Geometry check sheet. Reference: drawing and pictorial views, mm from the part's lowest x, y, z. A direction names the side the tool comes from. Give positions to 0.01 mm unless a question says otherwise; leave off trailing zeros. Write each loop counter-clockwise with the first axis right and the second up, starting at its lowest first coordinate (ties: lowest second). Pieces come first, ordered by that corner, then holes. Notation, with made-up numbers: (11.5, -18) -> (32.5, -18) arc R15 ccw to (32.5, -9) -> close; hole circle Ø1 at (19, 79). An arc over 180 degrees is marked (long way). Use a Markdown table: item, result. Add a question column.
1. Set-up check for the marked faces 4, 5 and 6: record each of +Z, -Z, +X, -X, +Y, -Y from which the full face is reachable in a straight line by a thin tool's end or side.
2. Cross-section at D-D (y = 5.5). Count the separate pieces of the cut face and the enclosed holes in it, then the cut area to 3 significant figures.
3. Release check for a two-part mould opening along X. For the marked faces 1, 2 and 3 record: released by +X, released by -X, zero draft, split by the parting line, or undercut.
4. Cross-section at C-C (x = 11). Enter the section's corners in (y, z), then the cut area to 3 significant figures.
5. Scan lines: probe 1 along X at (y, z) = (2, 1.5); probe 2 along Z at (x, y) = (44, 14.25); probe 3 along Y at (x, z) = (8, 13). Record each from-to range of solid material in increasing order. Write a range as [from, to].
6. Cross-section at A-A (z = 11). Enter the section's corners in (x, y).
7. Cross-section at B-B (y = 12.25). Enter the section's corners in (x, z).
8. Gauge pin test, flat ends, axial feed: P1, Ø7, axis at x = 23.38, z = 10.99, coming from the +Y side; P2, Ø2.5, axis at y = 15.5, z = 11.5, coming from the -X side; P3, Ø1.5, axis at x = 13, y = 17, coming from the +Z side. Record the tip position at first contact, or that the pin passes through.
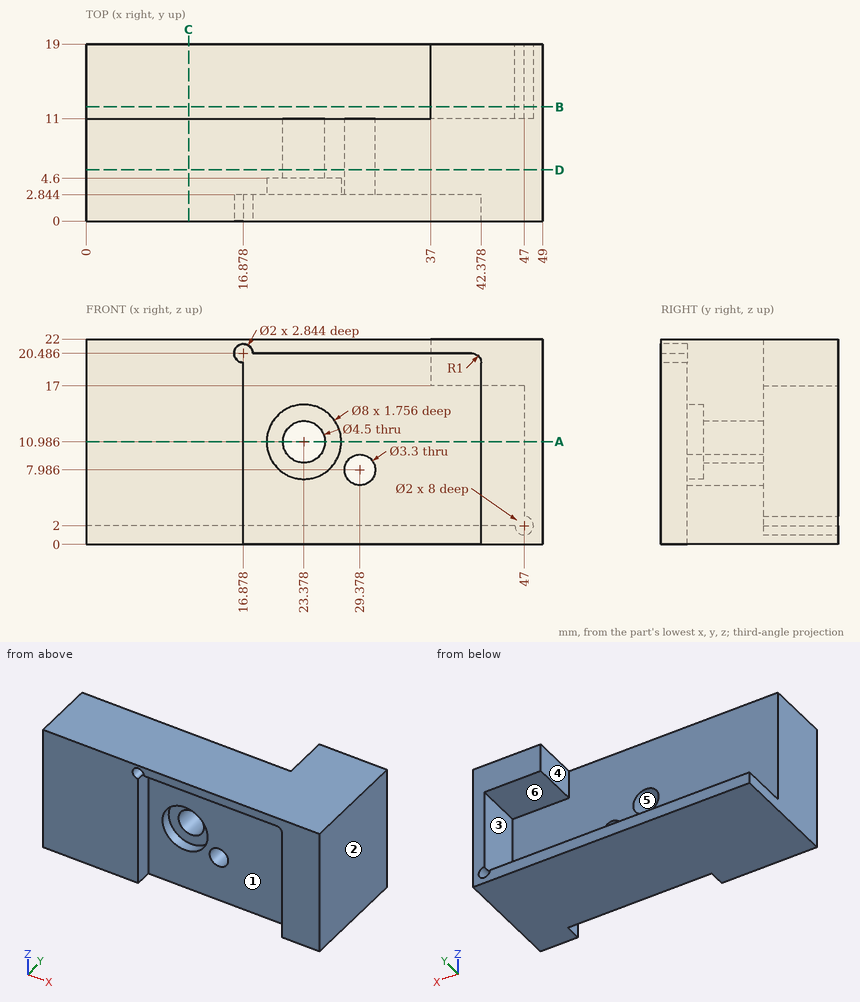
Worked answers:
| question | item | result |
|---|---|---|
| 1 | face 4 | +Z, -X, +Y |
| 1 | face 5 | +Y, -Y |
| 1 | face 6 | -X, +Y |
| 2 | separate pieces | 1 |
| 2 | enclosed holes | 2 |
| 2 | area | 1,050 mm² |
| 3 | face 1 | undercut |
| 3 | face 2 | released by +X |
| 3 | face 3 | released by -X |
| 4 | outline | (0, 0) -> (19, 0) -> (19, 2) -> (11, 2) -> (11, 22) -> (0, 22) -> close |
| 4 | area | 258 mm² |
| 5 | probe 1 | x = [0, 16.88], [42.38, 49] |
| 5 | probe 2 | z = [0, 2], [17, 22] |
| 5 | probe 3 | y = [0, 11] |
| 6 | outline | (0, 0) -> (16.88, 0) -> (16.88, 2.84) -> (19.38, 2.84) -> (19.38, 4.6) -> (21.13, 4.6) -> (21.13, 11) -> (0, 11) -> close; (25.63, 4.6) -> (27.38, 4.6) -> (27.38, 2.84) -> (42.38, 2.84) -> (42.38, 0) -> (49, 0) -> (49, 19) -> (47, 19) -> (47, 11) -> (25.63, 11) -> close |
| 7 | outline | (0, 0) -> (49, 0) -> (49, 22) -> (37, 22) -> (37, 17) -> (47, 17) -> (47, 3) arc R1 cw (long way) to (46, 2) -> (0, 2) -> close |
| 8 | P1 | stops at y = 11 |
| 8 | P2 | stops at x = 47 |
| 8 | P3 | stops at z = 2 |
